Geometry: final body of the model. Coordinates: model frame, mm. A direction names the side the tool comes from. Round coordinates to 2 decimals unless told otherwise and drop trailing zeros. Write each loop counter-clockwise with the first axis right and the second up, starting at its lowest first coordinate (ties: lowest second). Pieces come first, ordered by that corner, then holes. Notation, with made-up numbers: M 75,67.5 L 124,67.5 A29 ccw 124,103.5 Z; hole C 8,-6.75 d3. An arc over 180 degrees is marked long. Answer as CSV lines item,"result". Start each with the question number.
Q1. Ray query, probe 1 along Y at (x, z) = (3.75, 20); probe 2 along Y at (x, z) = (5, 48); probe 3 along Z at (x, y) = (5, 5). Return the intervals inside material, ascending.
Q2. Mould query, pull axis Y, two halves, no side actions, for faces 5 (the cylindrical face through (6.08, 3.16, 15.42)), 6 (the cylindrical face through (6.08, 13.61, 14.13)), 7 (the flat face through (6, 10, 27)), 8 (the flat face through (0, -1, 18)). Classes: pulls with the +Y half, pulls with the -Y half, needs draft (parallel to the pull), parting line crosses it, or undercut.
Q3. First-contact query: pin 1 (2 mm diameter, centred on x = 6, y = 11, fed in from +Z); pin 2 (6 mm diameter, centred on y = 6.5, z = 27, fed in from +X); pin 3 (1.5 mm diameter, centred on x = 5, z = 11.5, fed in from +Y). Flat tips, straight axial feed; report the tip coordinate or a pass-through.
Q4. Reachability of faces 1 (the cylindrical face through (11, 12, 32)), 2 (the cylindrical face through (6.08, 9.63, 18.18)), 3 (the cylindrical face through (1, 12, 32)), 4 (the flat face through (6, 12, 34)) from +Z, -Z, +X, -X, +Y, -Y: full face, straight path, thin tool, end or side. Return the list, or none.
Q5. Section query C-C on y = 11.5. Output: boundary loops of the cut face in (x, z), and give its area (3 significant figures).
Q6. Section query D-D on z = 9.5. Output: boundary loops of the cut face in (x, y).
Q7. Section query A-A on z = 22. Output: boundary loops of the cut face in (x, y).
```python
from build123d import *

# Parameters (mm, degrees)
F0_W     = 6
F0_H     = 50
F1_DEPTH = 4
F3_DEPTH = 12
F4_R     = 4.99999
F5_R     = 5


# Not quite as in the source:
# - a fillet or chamfer is up to 0.001 mm smaller than in the source, because OpenCascade refuses the exact size


with BuildPart() as f1:
    # F0 (on Front) → F1 (new body)
    with BuildSketch(Plane.XZ):
        with Locations((9, 25)):
            Rectangle(F0_W, F0_H)
        with Locations((3, 25)):
            Rectangle(F0_W, F0_H)
    extrude(amount=F1_DEPTH)

    # F2 (on Right) → F3 (join)
    with BuildSketch(Plane.YZ):
        Polygon((0, 8), (0, 0), (14, 14), (14, 34), (10, 34), (10, 18), align=None)
    extrude(amount=F3_DEPTH)

    # F4 (radius 5 in the source; OpenCascade refuses exactly that, so slightly less here)
    f4_edges = [f1.edges().sort_by_distance(p)[0] for p in [
        (0, -2, 50),
        (12, -2, 50),
        (0, 12, 34),
        (12, 12, 34),
        (6, 10, 18),
        (6, 14, 14),
        (6, 0, 8),
    ]]
    fillet(f4_edges, radius=F4_R)

    # F5
    f5_edges = [f1.edges().sort_by_distance(p)[0] for p in [
        (6, 0, 0),
    ]]
    fillet(f5_edges, radius=F5_R)


solid = f1.part
```
Entries:
1,probe 1,"y = -4 to 0, 10 to 14"
1,probe 2,"y = -4 to 0"
1,probe 3,"z = 5 to 15.07"
2,face 5,"undercut"
2,face 6,"pulls with the +Y half"
2,face 7,"undercut"
2,face 8,"needs draft"
3,pin 1,"stops at z = 34"
3,pin 2,"passes through"
3,pin 3,"stops at y = 12.25"
4,face 1,"+Z, +X, +Y"
4,face 2,"+Z, +X, -X"
4,face 3,"+Z, -X, +Y"
4,face 4,"+Z, +X, -X, +Y"
5,outline,"M 0,11.5 L 12,11.5 L 12,29 A5 ccw 7,34 L 5,34 A5 ccw 0,29 Z"
5,area,"259 mm^2"
6,outline,"M 0,-4 L 12,-4 L 12,9.5 L 0,9.5 Z"
7,outline,"M 0,-4 L 12,-4 L 12,0 L 0,0 Z; M 0,10 L 12,10 L 12,14 L 0,14 Z"
